```python
from build123d import *

# Parameters (mm, degrees)
SKETCH_W     = 50
SKETCH_H     = 35
PAD_DEPTH    = 10
SKETCH001_W  = 23.4
SKETCH001_H  = 23.4
POCKET_DEPTH = 10.001
FILLET_R     = 4
FILLET001_R  = 2


with BuildPart() as part:
    # Sketch → Pad (new body)
    with BuildSketch(Plane.XY):
        Rectangle(SKETCH_W, SKETCH_H)
    extrude(amount=PAD_DEPTH)

    # Sketch001 (on Face6 of Pad) → Pocket (cut, through all)
    with BuildSketch(Plane.XY.offset(10)):
        Rectangle(SKETCH001_W, SKETCH001_H)
    extrude(amount=-POCKET_DEPTH, mode=Mode.SUBTRACT)

    # Fillet
    fillet_edges = [part.edges().sort_by_distance(p)[0] for p in [
        (-25, 17.5, 5),
        (-25, -17.5, 5),
        (25, -17.5, 5),
        (25, 17.5, 5),
    ]]
    fillet(fillet_edges, radius=FILLET_R)

    # Fillet001
    fillet001_edges = [part.edges().sort_by_distance(p)[0] for p in [
        (-25, 0, 10),
        (-23.828427, 16.328427, 10),
        (0, 17.5, 10),
        (23.828427, 16.328427, 10),
        (25, 0, 10),
        (23.828427, -16.328427, 10),
        (0, -17.5, 10),
        (-23.828427, -16.328427, 10),
    ]]
    fillet(fillet001_edges, radius=FILLET001_R)


solid = part.part
```
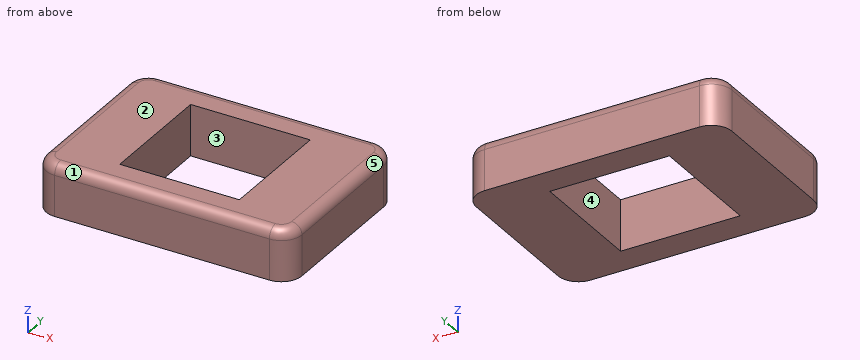
Check sheet for the modelled part. Datum: model origin and axes. Units: mm. Face numbers are marked on the shaded views. A direction names the side the tool comes from. Round coordinates to 2 decimals unless told otherwise and drop trailing zeros. Order: outer loops, then holes, each group sorted by start corner. A loop starts at its lowest first (then second) coordinate and runs counter-clockwise, first axis right, second up.
1) Scan lines: line 1 (X direction, y = 11, z = 5.25); line 2 (Y direction, x = -7.5, z = 6.5); line 3 (X direction, y = 7, z = 9.5). Record each from-to range of solid material in increasing order.
2) Tool access check on the marked faces 4 and 5. Record the directions out of +Z, -Z, +X, -X, +Y, -Y that give a thin tool (end or side, any length) a straight path to the whole face; none if there is none.
3) Section check A-A (y = -10). Record the boundary of the cut face in (x, z).
4) Section check B-B (x = 11). Record the boundary of the cut face in (y, z), and give its area (3 significant figures).
5) Section check C-C (z = 5). Record the boundary of the cut face in (x, y).
6) Mould release check, pull along Y, two halves, no side actions. Record for the marked faces 1, 2 and 3: +Y half, -Y half, draft (parallel to the pull), parting line (faces both ways), or undercut.
Result:
1. line 1: x = -25 to -11.7, 11.7 to 25
1. line 2: y = -17.5 to -11.7, 11.7 to 17.5
1. line 3: x = -24.32 to -11.7, 11.7 to 24.32
2. face 4: +Z, -Z
2. face 5: +Z, +X, +Y, -Y
3. outline: (-25, 0) - (-11.7, 0) - (-11.7, 10) - (-23, 10) arc R2 ccw to (-25, 8) - close; (11.7, 0) - (25, 0) - (25, 8) arc R2 ccw to (23, 10) - (11.7, 10) - close
4. outline: (-17.5, 0) - (-11.7, 0) - (-11.7, 10) - (-15.5, 10) arc R2 ccw to (-17.5, 8) - close; (11.7, 0) - (17.5, 0) - (17.5, 8) arc R2 ccw to (15.5, 10) - (11.7, 10) - close
4. area: 114 mm2
5. outline: (-25, -13.5) arc R4 ccw to (-21, -17.5) - (21, -17.5) arc R4 ccw to (25, -13.5) - (25, 13.5) arc R4 ccw to (21, 17.5) - (-21, 17.5) arc R4 ccw to (-25, 13.5) - close; hole (-11.7, -11.7) - (11.7, -11.7) - (11.7, 11.7) - (-11.7, 11.7) - close
6. face 1: -Y half
6. face 2: draft
6. face 3: undercut
